Geometry check sheet. Reference: the model listing, model coordinates, mm. A direction names the side the tool comes from. Coordinates: 2 decimals unless noted, no trailing zeros. Write each loop counter-clockwise with the first axis right and the second up, starting at its lowest first coordinate (ties: lowest second). Pieces come first, ordered by that corner, then holes. Notation, with made-up numbers: M -5,14.25 L 44,14.25 A11 ccw 44,35.25 Z; hole C 80,-33.5 d8. An arc over 180 degrees is marked long. Write each question's results on one line, items separated by ' | '.
```python
from build123d import *

# Parameters (mm, degrees)
SKETCH_1_W          = 36
SKETCH_1_H          = 21
SKETCH_1_R          = 1.25
SKETCH_1_R_2        = 1.3
SKETCH_1_R_3        = 1.35
EXTRUDE_1_DEPTH     = 30
SKETCH_1_5_R        = 1.3
SKETCH_1_5_R_2      = 1.35
SKETCH_1_5_R_3      = 1.25
CUT_EXTRUDE_1_DEPTH = 4
CUT_EXTRUDE_START   = 30
SKETCH_1_6_R        = 1.35
SKETCH_1_6_R_2      = 1.3
SKETCH_1_6_R_3      = 1.25
CUT_EXTRUDE_2_DEPTH = 4
CUT_EXTRUDE1_DEPTH  = 30


with BuildPart() as part:
    # 스케치1 → 보스-돌출1 (new body)
    with BuildSketch(Plane.XY):
        Rectangle(SKETCH_1_W, SKETCH_1_H)
        with Locations((-3.5, -8)):
            Circle(SKETCH_1_R, mode=Mode.SUBTRACT)
        with Locations((3.5, -8)):
            Circle(SKETCH_1_R, mode=Mode.SUBTRACT)
        with Locations((-12, 6)):
            Circle(SKETCH_1_R_2, mode=Mode.SUBTRACT)
        with Locations((12, 6)):
            Circle(SKETCH_1_R_2, mode=Mode.SUBTRACT)
        with Locations((12, -6)):
            Circle(SKETCH_1_R_2, mode=Mode.SUBTRACT)
        with Locations((-12, -6)):
            Circle(SKETCH_1_R_2, mode=Mode.SUBTRACT)
        with Locations((3.5, 8)):
            Circle(SKETCH_1_R_3, mode=Mode.SUBTRACT)
        with Locations((-3.5, 8)):
            Circle(SKETCH_1_R_3, mode=Mode.SUBTRACT)
        with Locations((12, -6)):
            Circle(SKETCH_1_R_2)
        with Locations((3.5, -8)):
            Circle(SKETCH_1_R)
        with Locations((-3.5, -8)):
            Circle(SKETCH_1_R)
        with Locations((-12, -6)):
            Circle(SKETCH_1_R_2)
        with Locations((-12, 6)):
            Circle(SKETCH_1_R_2)
        with Locations((-3.5, 8)):
            Circle(SKETCH_1_R_3)
        with Locations((3.5, 8)):
            Circle(SKETCH_1_R_3)
        with Locations((12, 6)):
            Circle(SKETCH_1_R_2)
    extrude(amount=EXTRUDE_1_DEPTH)

    # 스케치1<5> → 컷-돌출1 (cut)
    with BuildSketch(Plane.XY):
        with Locations((12, 6)):
            Circle(SKETCH_1_5_R)
        with Locations((3.5, 8)):
            Circle(SKETCH_1_5_R_2)
        with Locations((-3.5, 8)):
            Circle(SKETCH_1_5_R_2)
        with Locations((-12, 6)):
            Circle(SKETCH_1_5_R)
        with Locations((-12, -6)):
            Circle(SKETCH_1_5_R)
        with Locations(Location((-3.5, -8, 0), (0, 0, 180))):
            Circle(SKETCH_1_5_R_3)
        with Locations((3.5, -8)):
            Circle(SKETCH_1_5_R_3)
        with Locations((12, -6)):
            Circle(SKETCH_1_5_R)
    extrude(amount=CUT_EXTRUDE_1_DEPTH, mode=Mode.SUBTRACT)

    # 스케치1<6> → 컷-돌출2 (cut)
    with BuildSketch(Plane.XY.offset(CUT_EXTRUDE_START)):
        with Locations((3.5, 8)):
            Circle(SKETCH_1_6_R)
        with Locations((12, 6)):
            Circle(SKETCH_1_6_R_2)
        with Locations((-3.5, 8)):
            Circle(SKETCH_1_6_R)
        with Locations((-12, 6)):
            Circle(SKETCH_1_6_R_2)
        with Locations((-12, -6)):
            Circle(SKETCH_1_6_R_2)
        with Locations(Location((-3.5, -8, 0), (0, 0, 180))):
            Circle(SKETCH_1_6_R_3)
        with Locations((3.5, -8)):
            Circle(SKETCH_1_6_R_3)
        with Locations((12, -6)):
            Circle(SKETCH_1_6_R_2)
    extrude(amount=-CUT_EXTRUDE_2_DEPTH, mode=Mode.SUBTRACT)

    # Sketch2 → Cut-Extrude1 (cut)
    with BuildSketch(Plane(origin=(0, 10.5, 0), x_dir=(1, 0, 0), z_dir=(0, 1, 0))):
        with BuildLine():
            Line((-3.671911896, -8.172290791), (4.36058603, -8.172290791))
            ThreePointArc((4.36058603, -8.172290791), (11.649583923, -15.461288684), (4.36058603, -22.750286576))
            Line((4.36058603, -22.750286576), (-3.671911896, -22.750286576))
            ThreePointArc((-3.671911896, -22.750286576), (-10.960909789, -15.461288684), (-3.671911896, -8.172290791))
        make_face()
    extrude(amount=-CUT_EXTRUDE1_DEPTH, mode=Mode.SUBTRACT)


solid = part.part
```
Q1. Sectioned sample at C-C on x = 0. Record the cut outline in (y, z).
Geometry check:
outline: M -10.5,0 L 10.5,0 L 10.5,8.17 L -10.5,8.17 Z; M -10.5,22.75 L 10.5,22.75 L 10.5,30 L -10.5,30 Z
Q2. Sectioned sample at B-B on y = -8. Record the cut outline in (x, z), and give its area (3 significant figures).
Geometry check:
outline: M -18,0 L -4.75,0 L -4.75,4 L -2.25,4 L -2.25,0 L 2.25,0 L 2.25,4 L 4.75,4 L 4.75,0 L 18,0 L 18,30 L 4.75,30 L 4.75,26 L 2.25,26 L 2.25,30 L -2.25,30 L -2.25,26 L -4.75,26 L -4.75,30 L -18,30 Z; hole M -3.67,8.17 L 4.36,8.17 A7.29 ccw 4.36,22.75 L -3.67,22.75 A7.29 ccw Z | area: 756 mm2
Q3. Sectioned sample at A-A on z = 27.25. Give the number of separate pieces and of enclosed holes in the cut face, and give its area (3 significant figures).
Geometry check:
separate pieces: 1 | enclosed holes: 8 | area: 713 mm2
Q4. Access from +Z, -Z, +X, -X, +Y, -Y to the whole of each face (thin tool, end or side, straight path). Record for faces 4 (the cylindrical face through (4.655, -8.479, 1.972)), 5 (the flat face through (0, 0, 22.75)), 6 (the flat face through (-18, 0, 15)), 7 (the flat face through (0, 0, 0)), 8 (the flat face through (-12, -6, 26)).
Geometry check:
face 4: -Z | face 5: +Y, -Y | face 6: +Z, -Z, -X, +Y, -Y | face 7: -Z, +X, -X, +Y, -Y | face 8: +Z
Q5. Mould release check, pull along Z, two halves, no side actions. Record for faces 1 (the flat face through (-3, -8, 26)), 2 (the flat face through (0, 0, 8.172)), 3 (the flat face through (18, 0, 15)): pulls with the +Z half, pulls with the -Z half, needs draft (parallel to the pull), parting line crosses it, or undercut.
Geometry check:
face 1: pulls with the +Z half | face 2: undercut | face 3: needs draft
Q6. Sectioned sample at D-D on z = 12.75. Record the cut outline in (x, y), and give its area (3 significant figures).
Geometry check:
outline: M -18,-10.5 L -10.44,-10.5 L -10.44,10.5 L -18,10.5 Z; M 11.13,-10.5 L 18,-10.5 L 18,10.5 L 11.13,10.5 Z | area: 303 mm2
Q7. Depth check by flat-ended pin: P1, Ø2, axis at x = -3.5, y = -8, coming from the -Z side; P2, Ø1.6, axis at x = -3.5, y = 8, coming from the +Z side. Enter the tip coordinate at first touch or a pass-through.
Geometry check:
P1: stops at z = 4 | P2: stops at z = 26
Q8. Scan lines: probe 1 along Y at (x, z) = (3.5, 27.5); probe 2 along Y at (x, z) = (12, 1.4); probe 3 along X at (y, z) = (6.75, 15.75). Record each from-to range of solid material in increasing order.
Geometry check:
probe 1: y = -10.5 to -9.25, -6.75 to 6.65, 9.35 to 10.5 | probe 2: y = -10.5 to -7.3, -4.7 to 4.7, 7.3 to 10.5 | probe 3: x = -18 to -10.96, 11.64 to 18
